Design review of the part built by this model. Coordinates are the model's own, in mm. Coordinates: 2 decimals unless noted, no trailing zeros. Loops run counter-clockwise (first coordinate to the right, second up) from the corner with the lowest first, then second, coordinate; pieces in that order, holes last. Notation, with made-up numbers: (15, 31.25) - (29, 31.25) arc R25 ccw to (29, 53.25) - close; hole circle Ø6 at (35.25, 66). An arc over 180 degrees is marked (long way). Answer in a Markdown table with one row per item. Add a question column.
(1) To check wall thickness, follow L1, parallel to X at y = 12, z = 14; L2, parallel to Z at x = 377, y = 2.25. State the ranges of each line that lie inside material, in increasing order. Write a range as [from, to].
(2) We need section C-C, the plane x = 1271.5. Write out the cut boundary in (y, z), plus the area to 3 significant figures.
(3) We need section A-A, the plane z = 9.5. Write out the cut boundary in (x, y), plus the area to 3 significant figures.
(4) We need section B-B, the plane y = 10.5. Write out the cut boundary in (x, z), plus the area to 3 significant figures.
from build123d import *

# Parameters (mm, degrees)
SKETCH1_W           = 1828.8
SKETCH1_H           = 101.6
BOSS_EXTRUDE1_DEPTH = 12.7
CUT_EXTRUDE1_DEPTH  = 12.7


with BuildPart() as part:
    # Sketch1 → Boss-Extrude1 (new body)
    with BuildSketch(Plane(origin=(0, 0, 0), x_dir=(1, 0, 0), z_dir=(0, 1, 0))):
        with Locations((874.865206316, 17.108399093)):
            Rectangle(SKETCH1_W, SKETCH1_H)
    extrude(amount=BOSS_EXTRUDE1_DEPTH)

    # Sketch2 → Cut-Extrude1 (cut)
    with BuildSketch(Plane(origin=(0, 12.7, 0), x_dir=(1, 0, 0), z_dir=(0, 1, 0))):
        Polygon((341.465206316, -33.691600907), (189.065206316, -33.691600907), (189.065206316, 17.108399093), (493.865206316, 17.108399093), (493.865206316, -33.691600907), align=None)
        Polygon((1408.265206316, -33.691600907), (1255.865206316, -33.691600907), (1255.865206316, 17.108399093), (1560.665206316, 17.108399093), (1560.665206316, -33.691600907), align=None)
        Polygon((874.865206316, -33.691600907), (722.465206316, -33.691600907), (722.465206316, 17.108399093), (1027.265206316, 17.108399093), (1027.265206316, -33.691600907), align=None)
    extrude(amount=-CUT_EXTRUDE1_DEPTH, mode=Mode.SUBTRACT)


solid = part.part
Responses:
| question | item | result |
|---|---|---|
| 1 | L1 | x = [-39.53, 189.07], [493.87, 722.47], [1027.27, 1255.87], [1560.67, 1789.27] |
| 1 | L2 | z = [-67.91, -17.11] |
| 2 | outline | (0, -67.91) - (12.7, -67.91) - (12.7, -17.11) - (0, -17.11) - close |
| 2 | area | 645 mm2 |
| 3 | outline | (-39.53, 0) - (189.07, 0) - (189.07, 12.7) - (-39.53, 12.7) - close; (493.87, 0) - (722.47, 0) - (722.47, 12.7) - (493.87, 12.7) - close; (1027.27, 0) - (1255.87, 0) - (1255.87, 12.7) - (1027.27, 12.7) - close; (1560.67, 0) - (1789.27, 0) - (1789.27, 12.7) - (1560.67, 12.7) - close |
| 3 | area | 11,600 mm2 |
| 4 | outline | (-39.53, -67.91) - (1789.27, -67.91) - (1789.27, 33.69) - (1560.67, 33.69) - (1560.67, -17.11) - (1255.87, -17.11) - (1255.87, 33.69) - (1027.27, 33.69) - (1027.27, -17.11) - (722.47, -17.11) - (722.47, 33.69) - (493.87, 33.69) - (493.87, -17.11) - (189.07, -17.11) - (189.07, 33.69) - (-39.53, 33.69) - close |
| 4 | area | 139,000 mm2 |
